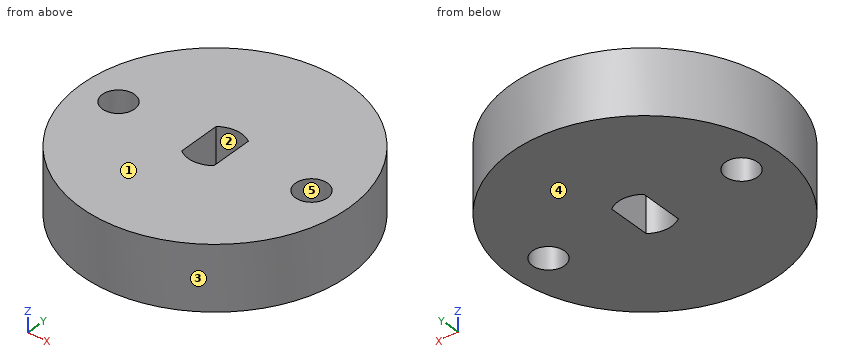
from build123d import *

# Parameters (mm, degrees)
SKETCH1_R           = 12.5
SKETCH1_R_2         = 1.5
BOSS_EXTRUDE1_DEPTH = 6


with BuildPart() as part:
    # Sketch1 → Boss-Extrude1 (new body)
    with BuildSketch(Plane.XY):
        Circle(SKETCH1_R)
        with BuildLine():
            Line((-1.5, -2), (-1.5, 2))
            ThreePointArc((-1.5, 2), (0, 2.5), (1.5, 2))
            Line((1.5, 2), (1.5, -2))
            ThreePointArc((1.5, -2), (0, -2.5), (-1.5, -2))
        make_face(mode=Mode.SUBTRACT)
        with Locations((-9, 0)):
            Circle(SKETCH1_R_2, mode=Mode.SUBTRACT)
        with Locations((9, 0)):
            Circle(SKETCH1_R_2, mode=Mode.SUBTRACT)
    extrude(amount=BOSS_EXTRUDE1_DEPTH)


solid = part.part
Design review of the part built by this model. Coordinates are the model's own, in mm. Face numbers are marked on the shaded views. A direction names the side the tool comes from. Coordinates: 2 decimals unless noted, no trailing zeros. Write each loop counter-clockwise with the first axis right and the second up, starting at its lowest first coordinate (ties: lowest second). Pieces come first, ordered by that corner, then holes. Notation, with made-up numbers: (-30, 28) - (23, 28) arc R13 cw to (23, 46) - close; hole circle Ø11 at (47, -29). An arc over 180 degrees is marked (long way). One line per item, written item: value.
1) Add section B-B (z = 3.2). State the section outline as (x, y) points, plus the area to 3 significant figures.
Answer sheet:
outline: circle Ø25 at (0, 0); hole circle Ø3 at (-9, 0); hole (-1.5, -2) arc R2.5 ccw to (1.5, -2) - (1.5, 2) arc R2.5 ccw to (-1.5, 2) - close; hole circle Ø3 at (9, 0)
area: 463 mm2
2) Add section A-A (x = 0). State the section outline as (y, z) points, plus the area to 3 significant figures.
Answer sheet:
outline: (-12.5, 0) - (-2.5, 0) - (-2.5, 6) - (-12.5, 6) - close; (2.5, 0) - (12.5, 0) - (12.5, 6) - (2.5, 6) - close
area: 120 mm2
3) Mouldability with a two-part tool opening along X and no side actions: class the marked faces 3, 4 and 5 as +X half, -X half, draft (parallel to the pull), parting line (faces both ways), or undercut.
Answer sheet:
face 3: parting line
face 4: draft
face 5: undercut
4) Insertion check: pin 1 (1.2 mm diameter, centred on y = -1, z = 1.5, fed in from -X); pin 2 (1 mm diameter, centred on x = 6, z = 4.5, fed in from -Y) (3 decimals); pin 3 (1.5 mm diameter, centred on y = 3, z = 0.5, fed in from -X); pin 4 (2.5 mm diameter, centred on x = -9, y = 0, fed in from +Z). Each pin has a flat end and moves straight along its axis. Give the tip position at first contact, or say it passes through.
Answer sheet:
pin 1: stops at x = -12.49
pin 2: stops at y = -11.225
pin 3: stops at x = -12.3
pin 4: passes through
5) To check wall thickness, follow probe 1 along X at (y, z) = (1.25, 2.4); probe 2 along X at (y, z) = (1.75, 5.55); probe 3 along Y at (x, z) = (-9, 2.65). State the ranges of each line that lie inside material, in increasing order.
Answer sheet:
probe 1: x = -12.44 to -9.83, -8.17 to -1.5, 1.5 to 8.17, 9.83 to 12.44
probe 2: x = -12.38 to -1.5, 1.5 to 12.38
probe 3: y = -8.67 to -1.5, 1.5 to 8.67
6) Add section D-D (x = 9). State the section outline as (y, z) points, plus the area to 3 significant figures.
Answer sheet:
outline: (-8.67, 0) - (-1.5, 0) - (-1.5, 6) - (-8.67, 6) - close; (1.5, 0) - (8.67, 0) - (8.67, 6) - (1.5, 6) - close
area: 86.1 mm2
7) For the marked faces 1 and 2, list the 3-axis set-ups (+Z, -Z, +X, -X, +Y, -Y) from which the entire face can be reached by the end or side of a thin tool; tool diameter is ignored.
Answer sheet:
face 1: +Z, +X, -X, +Y, -Y
face 2: +Z, -Z
8) Add section C-C (y = 0). State the section outline as (x, z) points.
Answer sheet:
outline: (-12.5, 0) - (-10.5, 0) - (-10.5, 6) - (-12.5, 6) - close; (-7.5, 0) - (-1.5, 0) - (-1.5, 6) - (-7.5, 6) - close; (1.5, 0) - (7.5, 0) - (7.5, 6) - (1.5, 6) - close; (10.5, 0) - (12.5, 0) - (12.5, 6) - (10.5, 6) - close
